Model file for the job. Use its own axes, mm. A direction names the side the tool comes from. Coordinates: 2 decimals unless noted, no trailing zeros. Write each loop counter-clockwise with the first axis right and the second up, starting at its lowest first coordinate (ties: lowest second). Pieces come first, ordered by that corner, then holes. Notation, with made-up numbers: M 68,55 L 101,55 A30 ccw 101,77 Z; hole C -26,-30 d11. An arc over 180 degrees is marked long. Answer in a Markdown table with one row per item. Add a question column.
Autodesk Inventor part; units mm, degrees
ref_plane "YZ Plane" through (0, 0, 0) normal (1, 0, 0) x (0, 1, 0)
ref_plane "XZ Plane" through (0, 0, 0) normal (0, 1, 0) x (-1, 0, 0)
ref_plane "XY Plane" through (0, 0, 0) normal (0, 0, 1) x (1, 0, 0)
sketch "Эскиз1" plane through (0, 0, 0) normal (0, 0, 1) x (1, 0, 0)
  arc A0 (4, 0) -> (-4, 0) centre (0, 0) ccw
  arc A1 (-16.1, 0) -> (-20.9, 0) centre (-18.5, 0) ccw
  arc A2 (20.9, 0) -> (16.1, 0) centre (18.5, 0) ccw
  line L0 (-24, 0) -> (24, 0)
  line L1 (-20.8784, 4.9592) -> (-5.8378, 12.1725)
  line L2 (20.8784, 4.9592) -> (5.8378, 12.1725)
  arc A3 (-20.8784, 4.9592) -> (-24, 0) centre (-18.5, 0) ccw
  arc A4 (24, 0) -> (20.8784, 4.9592) centre (18.5, 0) ccw
  arc A5 (5.8378, 12.1725) -> (-5.8378, 12.1725) centre (0, 0) ccw
  dimension "d0" = 8
  dimension "d9" = 37
  dimension "d12" = 4.8
  dimension "d14" = 48
  dimension "d15" = 5.5
  dimension "d16" = 13.5
  dimension "d19" = 0
extrude "Выдавливание1" add sketch "Эскиз1" along normal blind 4.5 contours A0 L0 A1 A3 L1 A5 L2 A4 A2
mirror "Зеркальное отражение1" about plane through (-24, 0, 0) normal (0, -1, 0) of "Выдавливание1"
sketch "Эскиз2" plane through (0, 0, 4.5) normal (0, 0, 1) x (1, 0, 0)
  circle A0 centre (0, 0) radius 4
  circle A1 centre (0, 0) radius 13.25
  dimension "d23" = 8
  dimension "d24" = 26.5
extrude "Выдавливание2" add sketch "Эскиз2" along normal blind 4
sketch "Эскиз5" plane through (0, 0, 8.5) normal (0, 0, 1) x (1, 0, 0)
  circle A0 centre (0, 0) radius 6
  circle A1 centre (0, 0) radius 4
  dimension "d33" = 12
  dimension "d34" = 8
extrude "Выдавливание5" add sketch "Эскиз5" along normal blind 7.5
properties part number "KFL08"
1) Which spindle directions (+Z, -Z, +X, -X, +Y, -Y) get a long thin tool onto all of the face, cutting with end or side? Do faces 4 (the face through (6, -3, 8.5)), 5 (the face through (-1.42, -3.92, 16)). Say none if no direction does.
2) Slice it at B-B (y = -11). Give the cut face in (x, z).
3) Slice it at D-D (z = 7.5). Give the cut face in (x, y), then the cut area to 3 significant figures.
4) Flat gauge pins, fed straight in: pin 1 Ø6 at (x, z) = (0.5, 10.5) entering from +Y; pin 2 Ø4.5 at (x, y) = (18.5, 0) entering from -Z; pin 3 Ø1.5 at (y, z) = (6, 10) entering from +X; pin 4 Ø3 at (x, z) = (-11.5, 5.5) entering from +Y. Where does each tip first touch, or does it go through?
5) Slice it at C-C (x = -12). Give the cut face in (y, z).
6) Two-plate mould, pull along Y, no slides. Class faces 1 (the face through (5, 0, 0)), 2 (the face through (13.5, 8.5, 2.2)), 3 (the face through (16.102, -0.106, 2.218)): released by +Y, released by -Y, zero draft, split by the parting line, or undercut.
7) Slice it at A-A (x = 20). Give the cut face in (y, z).
8) Drill centre lines: probe 1 along X at (y, z) = (0, 1.4); probe 2 along Y at (x, z) = (0, 9.75); probe 3 along Z at (x, y) = (-5.5, 5.75). Where is each one in solid material? Low to high.
Ans:
| question | item | result |
|---|---|---|
| 1 | face 4 | +Z |
| 1 | face 5 | +Z, +X, -X, +Y, -Y |
| 2 | outline | M -8.28,0 L 8.28,0 L 8.28,4.5 L 7.39,4.5 L 7.39,8.5 L -7.39,8.5 L -7.39,4.5 L -8.28,4.5 Z |
| 3 | outline | C 0,0 d26.5; hole C 0,0 d8 |
| 3 | area | 501 mm2 |
| 4 | pin 1 | stops at y = 13.25 |
| 4 | pin 2 | passes through |
| 4 | pin 3 | stops at x = 2.9 |
| 4 | pin 4 | stops at y = 9.99 |
| 5 | outline | M -9.22,0 L 9.22,0 L 9.22,4.5 L 5.62,4.5 L 5.62,8.5 L -5.62,8.5 L -5.62,4.5 L -9.22,4.5 Z |
| 6 | face 1 | zero draft |
| 6 | face 2 | released by +Y |
| 6 | face 3 | undercut |
| 7 | outline | M -5.38,0 L -1.87,0 L -1.87,4.5 L -5.38,4.5 Z; M 1.87,0 L 5.38,0 L 5.38,4.5 L 1.87,4.5 Z |
| 8 | probe 1 | x = -24 to -20.9, -16.1 to -4, 4 to 16.1, 20.9 to 24 |
| 8 | probe 2 | y = -6 to -4, 4 to 6 |
| 8 | probe 3 | z = 0 to 8.5 |
